Can you work these out from the model? Positions are in its coordinate system, mm. Face numbers are marked on the shaded views. Round coordinates to 2 decimals unless told otherwise and drop trailing zeros. Order: outer loops, then holes, each group sorted by start corner. A loop starts at its lowest first (then second) coordinate and runs counter-clockwise, first axis right, second up.
Q1. We'd pull the mould along X, two halves only. Please class the marked faces 1, 2 and 3: pulls with the +X half, pulls with the -X half, needs draft (parallel to the pull), parting line crosses it, or undercut.
Q2. If we section it at B-B (x = -2.5): Please give me the cut outline in (y, z), plus the area to 4 significant figures.
Q3. If we section it at A-A (z = -4.25): Please give me the cut outline in (x, y), plus the area to 3 significant figures.
Q4. If we section it at C-C (y = 23.5): Please give me the cut outline in (x, z), plus the area to 3 significant figures.
Q5. Will these pins go through, and if not, where does the flat tip stop? P1, Ø6, axis at x = -2, y = -10, coming from the -Z side; P2, Ø9, axis at x = -1, y = 0, coming from the -Z side; P3, Ø3, axis at x = -6, z = 0.5, coming from the -Y side.
Q6. If I drill on line 1 (X direction, y = 20.5, z = -1.25); line 2 (Z direction, x = -4, y = 12.5); line 3 (Y direction, x = 1, z = 1), over which ranges is the centre line in solid material (lowest first)?
from build123d import *

# Parameters (mm, degrees)
F0_R     = 1.5
F1_DEPTH = 2.5
F2_DEPTH = 8.5
F3_DEPTH = 1


with BuildPart() as f1:
    # F0 (on Top) → F1 (new body)
    with BuildSketch(Plane.XY):
        with BuildLine():
            Line((-3, -14.6969384567), (-3, 14.6969384567))
            ThreePointArc((-3, 14.6969384567), (-15, 0), (-3, -14.6969384567))
        make_face()
        with BuildLine():
            Line((3, -14.6969384567), (3, 14.6969384567))
            ThreePointArc((3, 14.6969384567), (0, 15), (-3, 14.6969384567))
            Line((-3, 14.6969384567), (-3, -14.6969384567))
            ThreePointArc((-3, -14.6969384567), (0, -15), (3, -14.6969384567))
        make_face()
        Circle(F0_R, mode=Mode.SUBTRACT)
        with BuildLine():
            ThreePointArc((3, -14.6969384567), (11.6189500386, -9.4868329805), (15, 0))
            ThreePointArc((15, 0), (11.6189500386, 9.4868329805), (3, 14.6969384567))
            Line((3, 14.6969384567), (3, -14.6969384567))
        make_face()
        with BuildLine():
            ThreePointArc((-3, 14.6969384567), (0, 15), (3, 14.6969384567))
            Line((3, 14.6969384567), (3, 27))
            ThreePointArc((3, 27), (2.1213203436, 29.1213203436), (0, 30))
            ThreePointArc((0, 30), (-2.1213203436, 29.1213203436), (-3, 27))
            Line((-3, 27), (-3, 14.6969384567))
        make_face()
        Circle(F0_R)
        Polygon((0.5773502692, 1), (0.8660253864, 0.5000000301), (1.1547005384, 0), (0.8660253864, -0.5000000301), (0.5773502692, -1), (0, -1), (-0.5773502692, -1), (-0.8660253838, -0.5000000347), (-1.1547005384, 0), (-0.866025389, 0.5000000256), (-0.5773502692, 1), (0, 1), align=None, mode=Mode.SUBTRACT)
    extrude(amount=F1_DEPTH)

    # F0 (on Top) → F2 (join)
    with BuildSketch(Plane.XY):
        with BuildLine():
            ThreePointArc((-3, 14.6969384567), (0, 15), (3, 14.6969384567))
            Line((3, 14.6969384567), (3, 27))
            ThreePointArc((3, 27), (2.1213203436, 29.1213203436), (0, 30))
            ThreePointArc((0, 30), (-2.1213203436, 29.1213203436), (-3, 27))
            Line((-3, 27), (-3, 14.6969384567))
        make_face()
    extrude(amount=-F2_DEPTH)

    # F0 (on Top) → F3 (join)
    with BuildSketch(Plane.XY):
        Circle(F0_R)
        Polygon((0.5773502692, 1), (0.8660253864, 0.5000000301), (1.1547005384, 0), (0.8660253864, -0.5000000301), (0.5773502692, -1), (0, -1), (-0.5773502692, -1), (-0.8660253838, -0.5000000347), (-1.1547005384, 0), (-0.866025389, 0.5000000256), (-0.5773502692, 1), (0, 1), align=None, mode=Mode.SUBTRACT)
    extrude(amount=-F3_DEPTH)


solid = f1.part
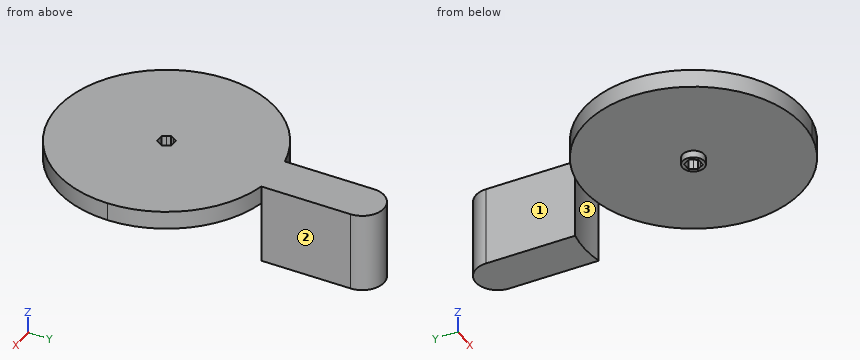
Solution:
1. face 1: pulls with the -X half
1. face 2: pulls with the +X half
1. face 3: undercut
2. outline: (-14.79, 0) - (14.79, 0) - (14.79, -8.5) - (28.66, -8.5) - (28.66, 2.5) - (-14.79, 2.5) - close
2. area: 226.5 mm2
3. outline: (-3, 14.7) arc R15 cw to (3, 14.7) - (3, 27) arc R3 ccw to (-3, 27) - close
3. area: 86.7 mm2
4. outline: (-3, -8.5) - (3, -8.5) - (3, 2.5) - (-3, 2.5) - close
4. area: 66.0 mm2
5. P1: stops at z = 0
5. P2: stops at z = -1
5. P3: stops at y = -14.31
6. line 1: x = -3 to 3
6. line 2: z = 0 to 2.5
6. line 3: y = -14.97 to -0.27, 0.27 to 29.83
